from build123d import *

# Parameters (mm, degrees)
SKETCH1_W                = 53.34
SKETCH1_H                = 24.5872
BOSS_EXTRUDE1_DEPTH      = 1.5875
SKETCH2_W                = 3.175
SKETCH2_H                = 2.38125
BOSS_EXTRUDE2_DEPTH      = 1.5875
BOSS_EXTRUDE2_2_DEPTH    = 1.5875
BOSS_EXTRUDE2_3_DEPTH    = 1.5875
LPATTERN1_COUNT          = 3
LPATTERN1_PITCH          = 15.24
BOSS_EXTRUDE3_DEPTH      = 9.525
BOSS_EXTRUDE3_DEPTH_BACK = 9.525
FILLET1_R                = 0.762


with BuildPart() as part:
    # Sketch1 → Boss-Extrude1 (new body)
    with BuildSketch(Plane(origin=(0, 0, 0), x_dir=(1, 0, 0), z_dir=(0, 1, 0))):
        with Locations((26.67, 12.2936)):
            Rectangle(SKETCH1_W, SKETCH1_H)
    extrude(amount=BOSS_EXTRUDE1_DEPTH)



with BuildPart() as body_2:
    # Sketch2 → Boss-Extrude2 (new body)
    with BuildSketch(Plane.XZ):
        with Locations((11.43, 1.190625)):
            Rectangle(SKETCH2_W, SKETCH2_H)
    extrude(amount=BOSS_EXTRUDE2_DEPTH)


with BuildPart() as body_3:
    # Sketch2 → Boss-Extrude2 2 (new body)
    with BuildSketch(Plane.XZ):
        with Locations((26.67, 1.190625)):
            Rectangle(SKETCH2_W, SKETCH2_H)
    extrude(amount=BOSS_EXTRUDE2_2_DEPTH)


with BuildPart() as body_4:
    # Sketch2 → Boss-Extrude2 3 (new body)
    with BuildSketch(Plane.XZ):
        with Locations((41.91, 1.190625)):
            Rectangle(SKETCH2_W, SKETCH2_H)
    extrude(amount=BOSS_EXTRUDE2_3_DEPTH)


with BuildPart() as part_1:
    add(part.part)

    add(body_4.part)  # Loft2 merges body 4
    # Sketch5 → Loft2 section 0
    with BuildSketch(Plane.XZ):
        with BuildLine():
            Line((37.1475, 0), (46.6725, 0))
            Line((46.6725, 0), (46.6725, -6.35))
            Line((46.6725, -6.35), (37.1475, -6.35))
            Line((37.1475, -6.35), (37.1475, 0))
        make_face()
    # Sketch4 → Loft2 section 1
    with BuildSketch(Plane.XZ.offset(1.5875)):
        with BuildLine():
            Line((43.4975, 0), (40.3225, 0))
            Line((40.3225, 0), (40.3225, -3.175))
            Line((40.3225, -3.175), (43.4975, -3.175))
            Line((43.4975, -3.175), (43.4975, 0))
        make_face()
    loft2 = loft()


    add(body_2.part)  # LPattern1 merges body 2

    add(body_3.part)  # LPattern1 merges body 3
    # LPattern1: Loft2 ×3
    with Locations(*[(-i * LPATTERN1_PITCH, 0, 0) for i in range(1, LPATTERN1_COUNT)]):
        add(loft2)

    # Sketch7 → Boss-Extrude3 (add, two sides: drawn at the far end of the back side and taken through both)
    with BuildSketch(Plane.ZY.offset(-26.67).offset(-BOSS_EXTRUDE3_DEPTH_BACK)):
        Polygon((-30.14345, -0.396875), (-28.55595, -1.984375), (-28.55595, -4.7625), (-26.212479769, -4.7625), (-24.5872, -4.7625), (-24.5872, 1.5875), (-25.38095, 1.5875), (-25.38095, -3.96875), (-27.7622, -3.96875), (-27.7622, 4.7625), (-28.55595, 4.7625), (-28.55595, 0), (-30.14345, 0), align=None)
    extrude(amount=BOSS_EXTRUDE3_DEPTH + BOSS_EXTRUDE3_DEPTH_BACK)

    # Fillet1
    fillet1_edges = [part_1.edges().sort_by_distance(p)[0] for p in [
        (26.67, -3.96875, -27.7622),
        (26.67, -3.96875, -25.38095),
        (26.67, 1.5875, -25.38095),
        (26.67, -4.7625, -24.5872),
        (26.67, -4.7625, -28.55595),
    ]]
    fillet(fillet1_edges, radius=FILLET1_R)


solid = part_1.part
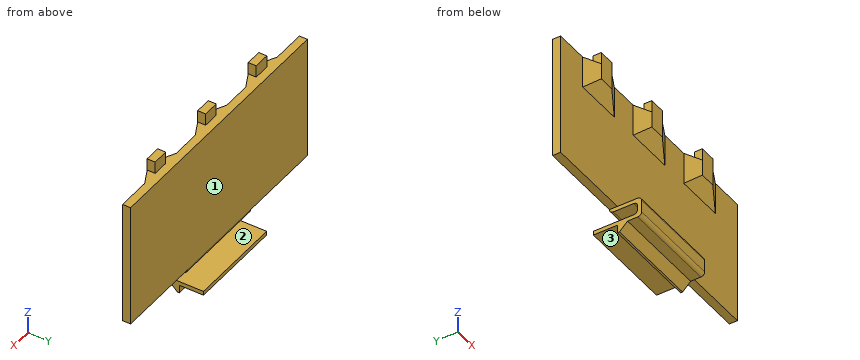
For this review, take the finished solid that the model builds, in its own axes (mm). Face numbers are marked on the shaded views. Round coordinates to 2 decimals unless told otherwise and drop trailing zeros. Order: outer loops, then holes, each group sorted by start corner. A loop starts at its lowest first (then second) coordinate and runs counter-clockwise, first axis right, second up. Notation, with made-up numbers: (-18, 22.5) -> (18, 22.5) arc R3 cw to (18, 27.5) -> close; hole circle Ø11 at (-23, -8.75). An arc over 180 degrees is marked (long way). Put each result on its own line as item: value.
Q1. Add section B-B on z = -17.5. Write out the cut boundary in (x, y).
Check result:
outline: (0, 0) -> (53.34, 0) -> (53.34, 1.59) -> (0, 1.59) -> close
Q2. Insertion check: pin 1 Ø2.5 at (x, y) = (26.5, 2.5) entering from -Z; pin 2 Ø0.5 at (x, z) = (27.5, -29.5) entering from +Y; pin 3 Ø0.5 at (y, z) = (-0.5, 1) entering from +X; pin 4 Ø10 at (x, z) = (18.5, -20.5) entering from -Y. Each pin has a flat end and moves straight along its axis. Give the tip position at first contact, or say it passes through.
Check result:
pin 1: z = -28.56
pin 2: y = 0
pin 3: x = 43.5
pin 4: y = -4.76
Q3. Add section C-C on y = -1. State how many separate pieces and enclosed holes the cut face has, plus the area to 3 significant figures.
Check result:
separate pieces: 5
enclosed holes: 0
area: 144 mm2
Q4. Mouldability with a two-part tool opening along Z and no side actions: class the marked faces 1, 2 and 3 as pulls with the +Z half, pulls with the -Z half, needs draft (parallel to the pull), parting line crosses it, or undercut.
Check result:
face 1: needs draft
face 2: undercut
face 3: pulls with the -Z half
Q5. Add section D-D on y = 4.25. Write out the cut boundary in (x, z) (3 decimals), plus the area to 3 significant figures.
Check result:
outline: (17.145, -28.556) -> (36.195, -28.556) -> (36.195, -27.762) -> (17.145, -27.762) -> close
area: 15.1 mm2
Q6. For probe 1 along Z at (x, y) = (33, -3.25); probe 2 along Y at (x, z) = (22.5, -7); probe 3 along Z at (x, y) = (42.5, 0.75), list the stretches that pass through material, from the lowest coordinate up. Write a range as [from, to].
Check result:
probe 1: [-28.56, -27.76], [-25.38, -24.59]
probe 2: [0, 1.59]
probe 3: [-24.59, 0]
Q7. Add section A-A on x = 34. Write out the cut boundary in (y, z), plus the area to 3 significant figures.
Check result:
outline: (-4.76, -27.79) arc R0.76 ccw to (-4, -28.56) -> (-1.98, -28.56) -> (-0.4, -30.14) -> (0, -30.14) -> (0, -28.56) -> (4.76, -28.56) -> (4.76, -27.76) -> (-3.21, -27.76) arc R0.76 cw to (-3.97, -27) -> (-3.97, -26.14) arc R0.76 cw to (-3.21, -25.38) -> (0.83, -25.38) arc R0.76 ccw to (1.59, -24.62) -> (1.59, 0) -> (0, 0) -> (0, -24.59) -> (-4, -24.59) arc R0.76 ccw to (-4.76, -25.35) -> close
area: 55.3 mm2
